Geometry check sheet. Reference: the model listing, model coordinates, mm. A direction names the side the tool comes from. Round coordinates to 2 decimals unless told otherwise and drop trailing zeros. Loops run counter-clockwise (first coordinate to the right, second up) from the corner with the lowest first, then second, coordinate; pieces in that order, holes last. Notation, with made-up numbers: (45, 29) - (64, 29) arc R29 cw to (64, 55) - close; hole circle Ø3 at (21, -21). An arc over 180 degrees is marked (long way). Answer as CSV lines item,"result". Start each with the question number.
1) Cross-section at A-A on x = 5. Record the boundary of the cut face in (y, z).
2) Thickness scan on line 1 along X through (y, z) = (7.75, 1); line 2 along X through (y, z) = (6.5, -20) (3 decimals); line 3 along Z through (x, y) = (-14, 2.5). Record the ranges inside material, lowest first.
3) Cross-section at C-C on z = -19. Record the boundary of the cut face in (x, y) (3 decimals).
4) Cross-section at B-B on y = 7. State how many separate pieces and enclosed holes the cut face has, and give its area (3 significant figures).
5) Draft check along X on faces 1 (the cylindrical face through (24.73, 4.93, 2.48)), 2 (the flat face through (-39.25, 5, 0)), 3 (the flat face through (-3, 5, 25)). Enter one of: released by +X, released by -X, zero draft, split by the parting line, or undercut.
6) Depth check by flat-ended pin: P1, Ø3, axis at y = 2, z = 25, coming from the -X side; P2, Ø0.5, axis at x = -21.5, z = -24, coming from the +Y side; P3, Ø5, axis at x = -7, y = 8, coming from the +Z side. Enter the tip coordinate at first touch or a pass-through.
7) Access from +Z, -Z, +X, -X, +Y, -Y to the whole of each face (thin tool, end or side, straight path). Record for faces 4 (the cylindrical face through (-22.72, 5.07, -4.25)), 5 (the flat face through (0, 0.8, 27.3)), 6 (the flat face through (-25.475, 6, -20)), 7 (the flat face through (3.5, 2, 25)).
from build123d import *

# Parameters (mm, degrees)
SKETCH1_R           = 1.925
BOSS_EXTRUDE1_DEPTH = 10
SKETCH2_R           = 11.25
SKETCH2_R_2         = 1.65
CUT_EXTRUDE1_DEPTH  = 49.845189118
SKETCH7_W           = 46
SKETCH7_H           = 4.1
CUT_EXTRUDE6_DEPTH  = 5
SKETCH10_W          = 4.6
SKETCH10_H          = 10
CUT_EXTRUDE8_DEPTH  = 10
CUT_EXTRUDE7_DEPTH  = 49.845189118
SKETCH13_W          = 7
SKETCH13_H          = 5
BOSS_EXTRUDE2_DEPTH = 1
CUT_EXTRUDE9_DEPTH  = 8.95
FILLET7_R           = 0.5
CUT_EXTRUDE10_DEPTH = 49.845189118
FILLET8_R           = 0.5
FILLET9_R           = 1.5


with BuildPart() as part:
    # Sketch1 → Boss-Extrude1 (new body)
    with BuildSketch(Plane(origin=(0, 0, 0), x_dir=(1, 0, 0), z_dir=(0, 1, 0))):
        Polygon((16, -23.2), (3.5, -23.2), (3.5, -27.3), (-3.5, -27.3), (-3.5, -23.2), (-16, -23.2), (-16, -27.3), (-23, -27.3), (-23, -23.2), (-39.25, -23.2), (-39.25, 23.2), (-23, 23.2), (23, 23.2), (27.25, 23.2), (27.25, -23.2), (23, -23.2), (23, -27.3), (16, -27.3), align=None)
        with Locations(Location((2, -15, 0), (0, 0, 270))):
            Circle(SKETCH1_R, mode=Mode.SUBTRACT)
        with Locations(Location((2, 15, 0), (0, 0, 270))):
            Circle(SKETCH1_R, mode=Mode.SUBTRACT)
    extrude(amount=BOSS_EXTRUDE1_DEPTH)

    # Sketch2 → Cut-Extrude1 (cut, through all)
    with BuildSketch(Plane(origin=(0, 10, 0), x_dir=(1, 0, 0), z_dir=(0, 1, 0))):
        with Locations(Location((0, 0, 0), (0, 0, 270))):
            Circle(SKETCH2_R)
        with Locations(Location((-15.5, 15.5, 0), (0, 0, 270))):
            Circle(SKETCH2_R_2)
        with Locations(Location((15.5, 15.5, 0), (0, 0, 270))):
            Circle(SKETCH2_R_2)
        with Locations(Location((15.5, -15.5, 0), (0, 0, 270))):
            Circle(SKETCH2_R_2)
        with Locations(Location((-15.5, -15.5, 0), (0, 0, 270))):
            Circle(SKETCH2_R_2)
    extrude(amount=-CUT_EXTRUDE1_DEPTH, mode=Mode.SUBTRACT)

    # Sketch7 → Cut-Extrude6 (cut)
    with BuildSketch(Plane(origin=(0, 10, 0), x_dir=(1, 0, 0), z_dir=(0, 1, 0))):
        with Locations((0, -25.25)):
            Rectangle(SKETCH7_W, SKETCH7_H)
    extrude(amount=-CUT_EXTRUDE6_DEPTH, mode=Mode.SUBTRACT)

    # Sketch10 → Cut-Extrude8 (cut)
    with BuildSketch(Plane(origin=(0, 10, 0), x_dir=(1, 0, 0), z_dir=(0, 1, 0))):
        with Locations((-34.45, 10)):
            Rectangle(SKETCH10_W, SKETCH10_H)
        with Locations((-34.45, -10)):
            Rectangle(SKETCH10_W, SKETCH10_H)
        with Locations((22.45, 7.5)):
            Rectangle(SKETCH10_W, SKETCH10_H)
        with Locations((22.45, -7.5)):
            Rectangle(SKETCH10_W, SKETCH10_H)
    extrude(amount=-CUT_EXTRUDE8_DEPTH, mode=Mode.SUBTRACT)

    # Sketch8 → Cut-Extrude7 (cut, through all)
    with BuildSketch(Plane.XZ):
        with BuildLine():
            Line((-23, 23.2), (-23, 27.3))
            ThreePointArc((-23, 27.3), (-24.5, 28.8), (-26, 27.3))
            Line((-26, 27.3), (-26, 23.2))
            ThreePointArc((-26, 23.2), (-24.5, 21.7), (-23, 23.2))
        make_face()
        with BuildLine():
            Line((13, 23.2), (13, 27.3))
            ThreePointArc((13, 27.3), (14.5, 28.8), (16, 27.3))
            Line((16, 27.3), (16, 23.2))
            ThreePointArc((16, 23.2), (14.5, 21.7), (13, 23.2))
        make_face()
        with BuildLine():
            Line((6.5, 27.3), (6.5, 23.2))
            ThreePointArc((6.5, 23.2), (5, 21.7), (3.5, 23.2))
            Line((3.5, 23.2), (3.5, 27.3))
            ThreePointArc((3.5, 27.3), (5, 28.8), (6.5, 27.3))
        make_face()
        with BuildLine():
            Line((-13, 23.2), (-13, 27.3))
            ThreePointArc((-13, 27.3), (-14.5, 28.8), (-16, 27.3))
            Line((-16, 27.3), (-16, 23.2))
            ThreePointArc((-16, 23.2), (-14.5, 21.7), (-13, 23.2))
        make_face()
        with BuildLine():
            Line((-6.5, 27.3), (-6.5, 23.2))
            ThreePointArc((-6.5, 23.2), (-5, 21.7), (-3.5, 23.2))
            Line((-3.5, 23.2), (-3.5, 27.3))
            ThreePointArc((-3.5, 27.3), (-5, 28.8), (-6.5, 27.3))
        make_face()
        with BuildLine():
            ThreePointArc((22.45, 12.284346805), (25.189339828, 11.439339828), (22.45, 10.594332852))
            ThreePointArc((22.45, 10.594332852), (19.710660172, 11.439339828), (22.45, 12.284346805))
        make_face()
        with BuildLine():
            ThreePointArc((22.45, 2.715653195), (25.189339828, 3.560660172), (22.45, 4.405667148))
            ThreePointArc((22.45, 4.405667148), (19.710660172, 3.560660172), (22.45, 2.715653195))
        make_face()
        with BuildLine():
            ThreePointArc((-34.45, -14.784346805), (-37.189339828, -13.939339828), (-34.45, -13.094332852))
            ThreePointArc((-34.45, -13.094332852), (-31.710660172, -13.939339828), (-34.45, -14.784346805))
        make_face()
        with BuildLine():
            ThreePointArc((-34.45, -5.215653195), (-37.189339828, -6.060660172), (-34.45, -6.905667148))
            ThreePointArc((-34.45, -6.905667148), (-31.710660172, -6.060660172), (-34.45, -5.215653195))
        make_face()
        with BuildLine():
            ThreePointArc((-34.45, 14.784346805), (-31.710660172, 13.939339828), (-34.45, 13.094332852))
            ThreePointArc((-34.45, 13.094332852), (-37.189339828, 13.939339828), (-34.45, 14.784346805))
        make_face()
        with BuildLine():
            ThreePointArc((-34.45, 5.215653195), (-31.710660172, 6.060660172), (-34.45, 6.905667148))
            ThreePointArc((-34.45, 6.905667148), (-37.189339828, 6.060660172), (-34.45, 5.215653195))
        make_face()
        with BuildLine():
            ThreePointArc((22.45, -12.284346805), (19.710660172, -11.439339828), (22.45, -10.594332852))
            ThreePointArc((22.45, -10.594332852), (25.189339828, -11.439339828), (22.45, -12.284346805))
        make_face()
        with BuildLine():
            ThreePointArc((22.45, -2.715653195), (19.710660172, -3.560660172), (22.45, -4.405667148))
            ThreePointArc((22.45, -4.405667148), (25.189339828, -3.560660172), (22.45, -2.715653195))
        make_face()
    extrude(amount=-CUT_EXTRUDE7_DEPTH, mode=Mode.SUBTRACT)

    # Sketch13 → Boss-Extrude2 (add)
    with BuildSketch(Plane(origin=(0, 0, -23.2), x_dir=(-1, 0, 0), z_dir=(0, 0, -1))):
        with Locations((23.83, 2.5)):
            Rectangle(SKETCH13_W, SKETCH13_H)
    extrude(amount=BOSS_EXTRUDE2_DEPTH)

    # Sketch12 → Cut-Extrude9 (cut)
    with BuildSketch(Plane.XZ.offset(-10)):
        with BuildLine():
            Line((-25.475, -24.2), (-25.475, -15.85))
            ThreePointArc((-25.475, -15.85), (-23.825, -14.2), (-22.175, -15.85))
            Line((-22.175, -15.85), (-22.175, -24.2))
            ThreePointArc((-22.175, -24.2), (-23.825, -25.85), (-25.475, -24.2))
        make_face()
        with BuildLine():
            Line((1.65, 27.3), (1.65, 18.95))
            ThreePointArc((1.65, 18.95), (0, 17.3), (-1.65, 18.95))
            Line((-1.65, 18.95), (-1.65, 27.3))
            ThreePointArc((-1.65, 27.3), (0, 28.95), (1.65, 27.3))
        make_face()
    extrude(amount=CUT_EXTRUDE9_DEPTH, mode=Mode.SUBTRACT)

    # Fillet7
    fillet7_edges = [part.edges().sort_by_distance(p)[0] for p in [
        (-39.25, 5, 23.2),
        (-39.25, 5, -23.2),
        (27.25, 5, -23.2),
        (27.25, 5, 23.2),
        (-20.33, 2.5, -24.2),
        (-27.33, 2.5, -24.2),
        (-22.175, 3.025, -24.2),
        (-25.475, 3.025, -24.2),
        (-1.65, 3.025, 27.3),
        (1.65, 3.025, 27.3),
        (23, 2.5, 27.3),
        (16, 2.5, 27.3),
        (3.5, 2.5, 27.3),
        (-3.5, 2.5, 27.3),
        (-16, 2.5, 27.3),
        (-23, 2.5, 27.3),
    ]]
    fillet(fillet7_edges, radius=FILLET7_R)

    # Sketch14 → Cut-Extrude10 (cut, through all)
    with BuildSketch(Plane.XZ.offset(-10)):
        with BuildLine():
            Line((-21.25, 8.75), (-28.75, 8.75))
            Line((-28.75, 8.75), (-28.75, -8.75))
            ThreePointArc((-28.75, -8.75), (-28.310660172, -9.810660172), (-27.25, -10.25))
            Line((-27.25, -10.25), (-22.75, -10.25))
            ThreePointArc((-22.75, -10.25), (-21.689339828, -9.810660172), (-21.25, -8.75))
            Line((-21.25, -8.75), (-21.25, -5.75))
            ThreePointArc((-21.25, -5.75), (-22.75, -4.25), (-24.25, -5.75))
            Line((-24.25, -5.75), (-24.25, -7.25))
            Line((-24.25, -7.25), (-25.75, -7.25))
            Line((-25.75, -7.25), (-25.75, 1.25))
            Line((-25.75, 1.25), (-24.25, 1.25))
            Line((-24.25, 1.25), (-24.25, -0.25))
            ThreePointArc((-24.25, -0.25), (-22.75, -1.75), (-21.25, -0.25))
            Line((-21.25, -0.25), (-21.25, 8.75))
        make_face()
    extrude(amount=CUT_EXTRUDE10_DEPTH, mode=Mode.SUBTRACT)

    # Fillet8
    fillet8_edges = [part.edges().sort_by_distance(p)[0] for p in [
        (-25.75, 5, -7.25),
        (-25.75, 5, 1.25),
    ]]
    fillet(fillet8_edges, radius=FILLET8_R)

    # Fillet9
    fillet9_edges = [part.edges().sort_by_distance(p)[0] for p in [
        (-21.25, 5, 8.75),
        (-28.75, 5, 8.75),
    ]]
    fillet(fillet9_edges, radius=FILLET9_R)


solid = part.part
Answer block:
1,outline,"(0, -23.2) - (10, -23.2) - (10, -10.08) - (0, -10.08) - close; (0, 10.08) - (10, 10.08) - (10, 21.7) - (0, 21.7) - close"
2,line 1,"x = -39.25 to -28.75, -25.68 to -24.25, -21.25 to -11.21, 11.21 to 27.25"
2,line 2,"x = -39.25 to -25.475, -22.175 to 27.25"
2,line 3,"z = -23.2 to -16.19, -14.81 to 14.81, 16.19 to 21.79"
3,outline,"(-39.25, 0) - (27.25, 0) - (27.25, 10) - (-22.175, 10) - (-22.175, 1.05) - (-25.475, 1.05) - (-25.475, 10) - (-39.25, 10) - close"
4,separate pieces,"1"
4,enclosed holes,"12"
4,area,"2,240 mm^2"
5,face 1,"undercut"
5,face 2,"released by -X"
5,face 3,"zero draft"
6,P1,"stops at x = -23"
6,P2,"stops at y = 5"
6,P3,"stops at z = 23.2"
7,face 4,"+Y, -Y"
7,face 5,"+Z, +X, -X, +Y, -Y"
7,face 6,"-Z, +Y"
7,face 7,"+Z, +Y, -Y"
